Work out the finished part from the listing and answer in its coordinate system (mm). A direction names the side the tool comes from. Round coordinates to 2 decimals unless told otherwise and drop trailing zeros. Loops run counter-clockwise (first coordinate to the right, second up) from the corner with the lowest first, then second, coordinate; pieces in that order, holes last. Notation, with made-up numbers: (75.5, 62) - (102.5, 62) arc R27 cw to (102.5, 101) - close; hole circle Ø11 at (-11, -40). An arc over 180 degrees is marked (long way). Return JSON: item names as keys, results as strings.
from build123d import *

# Parameters (mm, degrees)
F0_W     = 88.9
F0_H     = 29.21
F0_W_2   = 82.55
F0_H_2   = 22.86
F1_DEPTH = 38.1
F2_W     = 9.525
F2_H     = 15.875
F3_DEPTH = 25.4
F5_DEPTH = 88.9
F6_R     = 3.302
F7_DEPTH = 88.901
F8_W     = 12.7
F8_H     = 22.225
F9_DEPTH = 29.211


with BuildPart() as f1:
    # F0 (on Top) → F1 (new body)
    with BuildSketch(Plane.XY):
        Rectangle(F0_W, F0_H)
        Rectangle(F0_W_2, F0_H_2, mode=Mode.SUBTRACT)
    extrude(amount=F1_DEPTH)

    # F2 (on face) → F3 (cut)
    with BuildSketch(Plane(origin=(-44.45, 0, 0), x_dir=(0, -1, 0), z_dir=(-1, 0, 0))):
        with Locations((0, 7.9375)):
            Rectangle(F2_W, F2_H)
    extrude(amount=-F3_DEPTH, mode=Mode.SUBTRACT)

    # F4 (on face) → F5 (join, through all)
    with BuildSketch(Plane.YZ.offset(44.45)):
        with BuildLine():
            Line((14.605, 38.1), (7.304389, 55.448618))
            ThreePointArc((7.304389, 55.448618), (0, 60.2996), (-7.304389, 55.448618))
            Line((-7.304389, 55.448618), (-14.605, 38.1))
            Line((-14.605, 38.1), (14.605, 38.1))
        make_face()
    extrude(amount=-F5_DEPTH)

    # F6 (on face) → F7 (cut, through all)
    with BuildSketch(Plane.YZ.offset(44.45)):
        with Locations((0, 52.3748)):
            Circle(F6_R)
    extrude(amount=-F7_DEPTH, mode=Mode.SUBTRACT)

    # F8 (on face) → F9 (cut, through all)
    with BuildSketch(Plane.XZ.offset(14.605)):
        with Locations((-25.4, 52.3875)):
            Rectangle(F8_W, F8_H)
        with Locations((0, 52.3875)):
            Rectangle(F8_W, F8_H)
        with Locations((25.4, 52.3875)):
            Rectangle(F8_W, F8_H)
    extrude(amount=-F9_DEPTH, mode=Mode.SUBTRACT)


solid = f1.part
1) Section A-A (x = -24.5) is taken. Give the vertices of the cut face in (y, z) (3 decimals).
Verdict:
{"outline": "(-14.605, 0) - (-11.43, 0) - (-11.43, 38.1) - (11.43, 38.1) - (11.43, 0) - (14.605, 0) - (14.605, 38.1) - (13.269, 41.275) - (-13.269, 41.275) - (-14.605, 38.1) - close"}
2) Flat-ended cylindrical pins translate along their axes: pin 1 (3 mm diameter, centred on x = -21, y = 9.5, fed in from -Z); pin 2 (14 mm diameter, centred on x = 26.5, y = -5, fed in from +Z); pin 3 (6.5 mm diameter, centred on x = -26.5, y = 6, fed in from +Z) (3 decimals); pin 4 (6 mm diameter, centred on y = 0, z = 52.37, fed in from -X). Find the tip coordinate at first contact, or state that the pin passes through.
Verdict:
{"pin 1": "stops at z = 38.1", "pin 2": "stops at z = 60.29", "pin 3": "stops at z = 41.275", "pin 4": "passes through"}
3) Determine the mould class of faces 4 (the flat face through (0, 12, 0)), 5 (the flat face through (-43, 4.762, 8)), 6 (the cylindrical face through (-38, 0.1, 60.3)) for opening direction Y: pulls with the +Y half, pulls with the -Y half, needs draft (parallel to the pull), parting line crosses it, or undercut.
Verdict:
{"face 4": "needs draft", "face 5": "undercut", "face 6": "parting line crosses it"}
4) A tool of negligible diameter and unlimited length cuts with its end or side. For faces 1 (the flat face through (-6.35, -0.2, 48.5)), 2 (the flat face through (-43, 0, 15.875)), 3 (the flat face through (41.275, 0, 19)), from which of +Z, -Z, +X, -X, +Y, -Y can it reach the whole face along a straight path? Write none if from no direction.
Verdict:
{"face 1": "+Z, +Y, -Y", "face 2": "-Z, -X", "face 3": "-Z"}
5) Section B-B (z = 27.5) is taken. Give the vertices of the cut face in (x, y) (3 decimals), and give its area (3 significant figures).
Verdict:
{"outline": "(-44.45, -14.605) - (44.45, -14.605) - (44.45, 14.605) - (-44.45, 14.605) - close; hole (-41.275, -11.43) - (41.275, -11.43) - (41.275, 11.43) - (-41.275, 11.43) - close", "area": "710 mm2"}
6) Find the intervals of material crossed by L1, parallel to X at y = -10, z = 47; L2, parallel to Y at x = -15, z = 9 (3 decimals), in increasing order.
Verdict:
{"L1": "x = -44.45 to -31.75, -19.05 to -6.35, 6.35 to 19.05, 31.75 to 44.45", "L2": "y = -14.605 to -11.43, 11.43 to 14.605"}
7) Section C-C (y = 0) is taken. Count the separate pieces of the cut face and the enclosed holes in it, and give its area (3 significant figures).
Verdict:
{"separate pieces": "5", "enclosed holes": "0", "area": "1,100 mm2"}
